```python
from build123d import *

# Parameters (mm, degrees)
F0_W        = 60
F0_H        = 85
F1_DEPTH    = 5
F3_DEPTH    = 85
F4_DEPTH    = 85
F5_T1_DEPTH = 85
F6_T1_DEPTH = 90.0557507085


# Not quite as in the source:
# - a fillet or chamfer that OpenCascade refuses, or shapes differently, is made with other operations: its cross-section is extruded or revolved along the edge and cut away or added


with BuildPart() as f1:
    # F0 (on Front) → F1 (new body)
    with BuildSketch(Plane.XZ):
        Rectangle(F0_W, F0_H)
    extrude(amount=F1_DEPTH)

    # F2 (on face) → F3 (join, through all)
    with BuildSketch(Plane.XY.offset(42.5)):
        with BuildLine():
            Line((-14.5279902258, -5), (-23.2163735325, -5))
            ThreePointArc((-23.2163735325, -5), (-39.9986276925, -27.1894659474), (-39.2300904919, -55))
            Line((-39.2300904919, -55), (-37.5641118623, -55))
            ThreePointArc((-37.5641118623, -55), (-36.1025868185, -25.3667283731), (-14.5279902258, -5))
        make_face()
        with BuildLine():
            Line((23.2163735325, -5), (14.5279902258, -5))
            ThreePointArc((14.5279902258, -5), (36.1025868185, -25.3667283731), (37.5641118623, -55))
            Line((37.5641118623, -55), (39.2300904919, -55))
            ThreePointArc((39.2300904919, -55), (39.9986276925, -27.1894659474), (23.2163735325, -5))
        make_face()
        with BuildLine():
            ThreePointArc((14.5279902258, -5), (0, -2.25), (-14.5279902258, -5))
            Line((-14.5279902258, -5), (14.5279902258, -5))
        make_face()
        with BuildLine():
            Line((14.5279902258, -5), (-14.5279902258, -5))
            ThreePointArc((-14.5279902258, -5), (-36.1025868185, -25.3667283731), (-37.5641118623, -55))
            Line((-37.5641118623, -55), (37.5641118623, -55))
            ThreePointArc((37.5641118623, -55), (36.1025868185, -25.3667283731), (14.5279902258, -5))
        make_face()
    extrude(amount=-F3_DEPTH)

    # F2 (on face) → F4 (cut, through all)
    with BuildSketch(Plane.XY.offset(42.5)):
        with BuildLine():
            Line((14.5279902258, -5), (-14.5279902258, -5))
            ThreePointArc((-14.5279902258, -5), (-36.1025868185, -25.3667283731), (-37.5641118623, -55))
            Line((-37.5641118623, -55), (37.5641118623, -55))
            ThreePointArc((37.5641118623, -55), (36.1025868185, -25.3667283731), (14.5279902258, -5))
        make_face()
        with BuildLine():
            ThreePointArc((14.5279902258, -5), (0, -2.25), (-14.5279902258, -5))
            Line((-14.5279902258, -5), (14.5279902258, -5))
        make_face()
    extrude(amount=-F4_DEPTH, mode=Mode.SUBTRACT)

    # F5: fillet of radius 3 on 2 edges, made by hand

    # F5_s2 → F5_t1 (join)
    with BuildSketch(Plane.XY.offset(-42.5)):
        with BuildLine():
            ThreePointArc((30, -5), (28.3606490054, -7.224664287), (29.2357538945, -9.8458842905))
            ThreePointArc((29.2357538945, -9.8458842905), (26.3377498383, -7.2842097229), (23.2163735325, -5))
            Line((23.2163735325, -5), (30, -5))
        make_face()
        with BuildLine():
            ThreePointArc((-29.2357538945, -9.8458842905), (-28.3606490054, -7.224664287), (-30, -5))
            Line((-30, -5), (-23.2163735325, -5))
            ThreePointArc((-23.2163735325, -5), (-26.3377498383, -7.2842097229), (-29.2357538945, -9.8458842905))
        make_face()
    extrude(amount=F5_T1_DEPTH)

    # F6: chamfer of 1 on 2 edges, made by hand

    # F6_s2 → F6_t1 (cut)
    with BuildSketch(Plane.XY.offset(-45.0278753542)):
        with BuildLine():
            Line((-37.8490587869, -54.0393279007), (-38.5747461473, -55.0322947503))
            Line((-38.5747461473, -55.0322947503), (-38.5747461473, -55.0522947503))
            ThreePointArc((-38.5747461473, -55.0522947503), (-38.0694290048, -55.02), (-37.5641118623, -55.02))
            Line((-37.5641118623, -55.02), (-37.5452116802, -54.9934591195))
            ThreePointArc((-37.5452116802, -54.9934591195), (-37.7059205116, -54.5194432134), (-37.8300033601, -54.0332541283))
            Line((-37.8300033601, -54.0332541283), (-37.8490587869, -54.0393279007))
        make_face()
        with BuildLine():
            Line((38.5747461473, -55.0322947503), (37.8490587869, -54.0393279007))
            Line((37.8490587869, -54.0393279007), (37.8300033601, -54.0332541283))
            ThreePointArc((37.8300033601, -54.0332541283), (37.7059205116, -54.5194432134), (37.5452116802, -54.9934591195))
            Line((37.5452116802, -54.9934591195), (37.5641118623, -55.02))
            ThreePointArc((37.5641118623, -55.02), (38.0694290048, -55.02), (38.5747461473, -55.0522947503))
            Line((38.5747461473, -55.0522947503), (38.5747461473, -55.0322947503))
        make_face()
    extrude(amount=F6_T1_DEPTH, mode=Mode.SUBTRACT)


solid = f1.part
```
Here's how the part is built. I have some questions about the finished solid (model axes, mm). A direction names the side the tool comes from. Give positions to 0.01 mm unless a question says otherwise; leave off trailing zeros. Write each loop counter-clockwise with the first axis right and the second up, starting at its lowest first coordinate (ties: lowest second). Pieces come first, ordered by that corner, then holes.
(1) Will these pins go through, and if not, where does the flat tip stop? pin 1 (8 mm diameter, centred on y = -49.5, z = 9.5, fed in from +X); pin 2 (3 mm diameter, centred on y = -36.5, z = -6.5, fed in from +X); pin 3 (8 mm diameter, centred on y = -37.5, z = -33, fed in from +X); pin 4 (1.5 mm diameter, centred on y = -2.5, z = 16.5, fed in from +X).
Output values:
pin 1: stops at x = 41.64
pin 2: stops at x = 41.95
pin 3: stops at x = 42
pin 4: stops at x = 30
(2) Imagine slicing it at B-B, the plane y = -12. Write out the boundary of the cut face in (x, z).
Output values:
outline: (-31.3, -42.5) - (-26.08, -42.5) - (-26.08, 42.5) - (-31.3, 42.5) - close; (26.08, -42.5) - (31.3, -42.5) - (31.3, 42.5) - (26.08, 42.5) - close
(3) Thinking about a two-plate mould opening in Z: for faces 4 (the face through (-40.932, -30.589, 0.595)), 5 (the face through (0, -1, 42.5)), 6 (the face through (0, -1, -42.5)), which applies, pulls with the +Z half, pulls with the -Z half, needs draft (parallel to the pull), parting line crosses it, or undercut?
Output values:
face 4: needs draft
face 5: pulls with the +Z half
face 6: pulls with the -Z half
(4) On a 3-axis mill with a long thin cutter (end or side, diameter ignored), from which of +Z, -Z, +X, -X, +Y, -Y can I reach the whole of each face in a straight line? I mean faces 1 (the face through (-30, -2, -1)), 2 (the face through (41.08, -31.26, 0.59)), 3 (the face through (30, -2, -1)). Say none if no direction works.
Output values:
face 1: +Z, -Z, -X, +Y
face 2: +Z, -Z, +X
face 3: +Z, -Z, +X, +Y
(5) Imagine slicing it at C-C, the plane x = 0. Write out the boundary of the cut face in (y, z), and give its area (3 significant figures).
Output values:
outline: (-2.25, -42.5) - (0, -42.5) - (0, 42.5) - (-2.25, 42.5) - close
area: 191 mm2
(6) Imagine slicing it at A-A, the plane z = 3. Write out the boundary of the cut face in (x, y).
Output values:
outline: (-39.23, -55) - (-38.55, -55) - (-37.87, -54.07) arc R39.75 cw (long way) to (37.87, -54.07) - (38.55, -55) - (39.23, -55) arc R42 ccw to (29.24, -9.85) arc R3 cw to (30, -5) - (30, 0) - (-30, 0) - (-30, -5) arc R3 cw to (-29.24, -9.85) arc R42 ccw to start
(7) If I drill on L1, parallel to X at y = -23.5, z = 17; L2, parallel to X at y = -45, z = 8; L3, parallel to Y at x = -14.5, z = -10, over which ranges is the centre line in solid material (lowest first)?
Output values:
L1: x = -38.62 to -35.18, 35.18 to 38.62
L2: x = -41.7 to -39.64, 39.64 to 41.7
L3: y = -4.99 to 0
(8) Imagine slicing it at D-D, the plane y = -47.5. Write out the boundary of the cut face in (x, z).
Output values:
outline: (-41.32, -42.5) - (-39.37, -42.5) - (-39.37, 42.5) - (-41.32, 42.5) - close; (39.37, -42.5) - (41.32, -42.5) - (41.32, 42.5) - (39.37, 42.5) - close
